Could you check a few things on this model? Use its own coordinates, in mm. A direction names the side the tool comes from. Give positions to 0.01 mm unless a question says otherwise; leave off trailing zeros. Loops run counter-clockwise (first coordinate to the right, second up) from the corner with the lowest first, then second, coordinate; pieces in that order, holes last. Notation, with made-up numbers: M -8.75,56 L 15.25,56 A20 cw 15.25,65 Z; hole C 65,-13.75 d9. An arc over 180 degrees is marked long. Answer in a Markdown table with one row per item. Add a question column.
```python
from build123d import *

# Parameters (mm, degrees)
F0_W     = 50.8
F0_H     = 50.8
F1_DEPTH = 50.8
F2_R     = 12.7
F3_DEPTH = 25.4
F4_R     = 12.7
F5_DEPTH = 50.8
F6_W     = 25.4
F6_H     = 25.4
F7_DEPTH = 25.4


with BuildPart() as f1:
    # F0 (on Front) → F1 (new body)
    with BuildSketch(Plane.XZ):
        with Locations((-25.4, 25.4)):
            Rectangle(F0_W, F0_H)
    extrude(amount=F1_DEPTH)

    # F2 (on face) → F3 (join)
    with BuildSketch(Plane.XZ.offset(50.8)):
        with Locations((-25.4, 25.4)):
            Circle(F2_R)
    extrude(amount=F3_DEPTH)

    # F4 (on face) → F5 (cut)
    with BuildSketch(Plane(origin=(-50.8, 0, 0), x_dir=(0, -1, 0), z_dir=(-1, 0, 0))):
        with Locations((25.4, 25.4)):
            Circle(F4_R)
    extrude(amount=-F5_DEPTH, mode=Mode.SUBTRACT)

    # F6 (on face) → F7 (join)
    with BuildSketch(Plane(origin=(0, 0, 0), x_dir=(-1, 0, 0), z_dir=(0, 1, 0))):
        with Locations((25.4, 25.4)):
            Rectangle(F6_W, F6_H)
    extrude(amount=F7_DEPTH)


solid = f1.part
```
Item 1: If we mould it in two halves opening along Z, with no side actions, what happens to faces 5 (the face through (-31, -50.8, 37)), 6 (the face through (-25, 13, 38.1)), 7 (the face through (-26, -25, 0)), 8 (the face through (-25.756, -16.04, 33.983))? For each: +Z half, -Z half, draft (parallel to the pull), parting line (faces both ways), or undercut.
Item 2: Suppose I cut it at C-C (x = -8.5). List the corners of the cut face in (y, z) for me.
Item 3: Suppose I cut it at B-B (z = 25.4). List the corners of the cut face in (x, y) for me.
Item 4: For P1, Ø12.5, axis at y = 7, z = 22.5, coming from the +X side; P2, Ø23, axis at y = -25.4, z = 25.4, coming from the +X side; P3, Ø4, axis at x = -12.5, z = 6, coming from the +Y side; P4, Ø3, axis at y = -59.5, z = 30, coming from the +X side, each with a flat end and sliding along its axis, tell me the tip position at first contact or that it passes through.
Item 5: Suppose I cut it at D-D (y = -52.5). List the corners of the cut face in (x, z) for me, then the cut area to 3 significant figures.
Item 6: I need wall thicknesses on L1, parallel to Z at x = -27, y = -25.4; L2, parallel to X at y = 16.5, z = 25.5; L3, parallel to Y at x = -5, z = 3.5. Which ranges of each line are inside material? Lowest first, please.
Item 7: Suppose I cut it at A-A (y = -25.4). List the corners of the cut face in (x, z) for me.
Item 8: For faces 1 (the face through (-18.573, -63.322, 36.109)), 2 (the face through (-38.1, 13, 25)), 3 (the face through (-25, 13, 12.7)), 4 (the face through (-12.7, 13, 25)), which set-ups out of +Z, -Z, +X, -X, +Y, -Y let a thin tool reach every point of the face, with its end or its side?
Values found:
| question | item | result |
|---|---|---|
| 1 | face 5 | draft |
| 1 | face 6 | +Z half |
| 1 | face 7 | -Z half |
| 1 | face 8 | undercut |
| 2 | outline | M -50.8,0 L 0,0 L 0,50.8 L -50.8,50.8 Z; hole C -25.4,25.4 d25.4 |
| 3 | outline | M -50.8,-50.8 L -38.1,-50.8 L -38.1,-76.2 L -12.7,-76.2 L -12.7,-50.8 L 0,-50.8 L 0,-38.1 L -50.8,-38.1 Z; M -50.8,-12.7 L 0,-12.7 L 0,0 L -12.7,0 L -12.7,25.4 L -38.1,25.4 L -38.1,0 L -50.8,0 Z |
| 4 | P1 | x = -12.7 |
| 4 | P2 | through |
| 4 | P3 | y = 0 |
| 4 | P4 | x = -13.08 |
| 5 | outline | C -25.4,25.4 d25.4 |
| 5 | area | 507 mm² |
| 6 | L1 | 0 to 12.7, 38.1 to 50.8 |
| 6 | L2 | -38.1 to -12.7 |
| 6 | L3 | -50.8 to 0 |
| 7 | outline | M -50.8,0 L 0,0 L 0,12.7 L -50.8,12.7 Z; M -50.8,38.1 L 0,38.1 L 0,50.8 L -50.8,50.8 Z |
| 8 | face 1 | -Y |
| 8 | face 2 | +Z, -Z, -X, +Y |
| 8 | face 3 | -Z, +X, -X, +Y |
| 8 | face 4 | +Z, -Z, +X, +Y |
